Here's how the part is built. I have some questions about the finished solid (model axes, mm). A direction names the side the tool comes from. Give positions to 0.01 mm unless a question says otherwise; leave off trailing zeros. Loops run counter-clockwise (first coordinate to the right, second up) from the corner with the lowest first, then second, coordinate; pieces in that order, holes last.
Q1. Suppose I cut it at C-C (y = 10.5). List the corners of the cut face in (x, z) for me (3 decimals).
Q2. Thinking about a two-plate mould opening in X: for faces 1 (the face through (177.8, 9, 2)), 2 (the face through (-177.8, 9, 2)), 3 (the face through (-2, 9, 177.8)), 4 (the face through (-2, 9, -114.3)), which applies, pulls with the +X half, pulls with the -X half, needs draft (parallel to the pull), parting line crosses it, or undercut?
Q3. For faces 5 (the face through (-2, 9, -177.8)), 6 (the face through (-2, 9, 114.3)), which set-ups out of +Z, -Z, +X, -X, +Y, -Y let a thin tool reach every point of the face, with its end or its side?
Q4. I need wall thicknesses on probe 1 along Z at (x, y) = (0, 9.75); probe 2 along Z at (x, y) = (-29, 9.75). Which ranges of each line are inside material? Lowest first, please.
Q5. Suppose I cut it at B-B (z = 40). List the corners of the cut face in (x, y) for me, and give its area (3 significant figures).
Q6. Suppose I cut it at A-A (x = -78). List the corners of the cut face in (y, z) for me.
Q7. I'm going to push a flat-ended pin straight in: P1, Ø9, axis at x = 142.875, z = 0, coming from the +Y side. Where does the tip first touch, or does it pass through?
```python
from build123d import *

# Parameters (mm, degrees)
SKETCH1_W               = 355.6
SKETCH1_H               = 355.6
BOSS_EXTRUDE1_DEPTH     = 18.25625
F_1_4_CLEARANCE_HOLE1_D = 6.7564
SKETCH8_W               = 228.6
SKETCH8_H               = 228.6
CUT_EXTRUDE3_DEPTH      = 253.109045185
FILLET2_R               = 3.3782


with BuildPart() as part:
    # Sketch1 → Boss-Extrude1 (new body)
    with BuildSketch(Plane(origin=(0, 0, 0), x_dir=(1, 0, 0), z_dir=(0, 1, 0))):
        Rectangle(SKETCH1_W, SKETCH1_H)
    extrude(amount=BOSS_EXTRUDE1_DEPTH)

    # 1/4 Clearance Hole1 (through all)
    with Locations(Plane(origin=(0, 18.25625, 0), x_dir=(1, 0, 0), z_dir=(0, 1, 0))):
        with Locations((0, 142.875), (-142.875, 0), (0, -142.875), (142.875, 0)):
            Hole(F_1_4_CLEARANCE_HOLE1_D / 2)

    # Sketch8 → Cut-Extrude3 (cut, through all)
    with BuildSketch(Plane(origin=(0, 18.25625, 0), x_dir=(1, 0, 0), z_dir=(0, 1, 0))):
        Rectangle(SKETCH8_W, SKETCH8_H)
    extrude(amount=-CUT_EXTRUDE3_DEPTH, mode=Mode.SUBTRACT)

    # Fillet2
    fillet2_edges = [part.edges().sort_by_distance(p)[0] for p in [
        (-114.3, 9.128125, 114.3),
        (-114.3, 9.128125, -114.3),
        (114.3, 9.128125, -114.3),
        (114.3, 9.128125, 114.3),
    ]]
    fillet(fillet2_edges, radius=FILLET2_R)


solid = part.part
```
Solutions:
1. outline: (-177.8, -177.8) - (177.8, -177.8) - (177.8, 177.8) - (-177.8, 177.8) - close; hole circle Ø6.756 at (-142.875, 0); hole (-114.3, -110.922) arc R3.378 ccw to (-110.922, -114.3) - (110.922, -114.3) arc R3.378 ccw to (114.3, -110.922) - (114.3, 110.922) arc R3.378 ccw to (110.922, 114.3) - (-110.922, 114.3) arc R3.378 ccw to (-114.3, 110.922) - close; hole circle Ø6.756 at (0, -142.875); hole circle Ø6.756 at (0, 142.875); hole circle Ø6.756 at (142.875, 0)
2. face 1: pulls with the +X half
2. face 2: pulls with the -X half
2. face 3: needs draft
2. face 4: undercut
3. face 5: -Z, +X, -X, +Y, -Y
3. face 6: +Y, -Y
4. probe 1: z = -177.8 to -146.25, -139.5 to -114.3, 114.3 to 139.5, 146.25 to 177.8
4. probe 2: z = -177.8 to -114.3, 114.3 to 177.8
5. outline: (-177.8, 0) - (-114.3, 0) - (-114.3, 18.26) - (-177.8, 18.26) - close; (114.3, 0) - (177.8, 0) - (177.8, 18.26) - (114.3, 18.26) - close
5. area: 2,320 mm2
6. outline: (0, -177.8) - (18.26, -177.8) - (18.26, -114.3) - (0, -114.3) - close; (0, 114.3) - (18.26, 114.3) - (18.26, 177.8) - (0, 177.8) - close
7. P1: stops at y = 18.26
